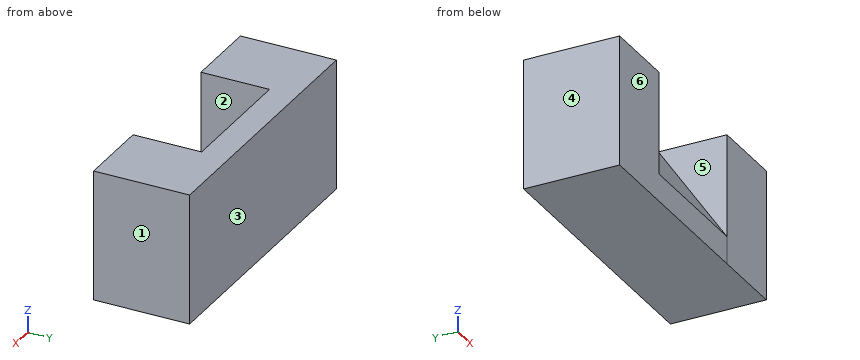
from build123d import *

# Parameters (mm, degrees)
F0_W     = 34.925
F0_H     = 60.325
F1_DEPTH = 44.45
F3_DEPTH = 60.325
F5_DEPTH = 34.925


with BuildPart() as f1:
    # F0 (on Front) → F1 (new body)
    with BuildSketch(Plane.XZ):
        with Locations((-46.881634, -30.1625)):
            Rectangle(F0_W, F0_H)
    extrude(amount=F1_DEPTH)

    # F2 (on face) → F3 (join)
    with BuildSketch(Plane.YZ.offset(-29.419134)):
        Polygon((-44.45, -47.625), (-44.45, -60.325), (0, -60.325), (0, -47.625), (0, 0), (-12.7, 0), align=None)
    extrude(amount=F3_DEPTH)

    # F4 (on face) → F5 (join)
    with BuildSketch(Plane.YZ.offset(30.905866)):
        Polygon((-44.45, -47.625), (-12.7, 0), (-44.459421, 0), (-44.45, -60.325), align=None)
        Polygon((0, -60.325), (0, 0), (-12.7, 0), (-44.45, -47.625), (-44.45, -60.325), align=None)
    extrude(amount=F5_DEPTH)


solid = f1.part
Design review of the part built by this model. Coordinates are the model's own, in mm. Face numbers are marked on the shaded views. A direction names the side the tool comes from. Round coordinates to 2 decimals unless told otherwise and drop trailing zeros. Loops run counter-clockwise (first coordinate to the right, second up) from the corner with the lowest first, then second, coordinate; pieces in that order, holes last. Notation, with made-up numbers: M 77.25,46 L 87.25,46 A23 ccw 87.25,72 Z; hole C -39.75,35.5 d2. An arc over 180 degrees is marked long. Answer as a JSON object with one key per item and string values.
Item 1: Clearance check with flat-ended pins moving along their axes: P1, Ø2, axis at x = 4, z = -51.5, coming from the -Y side; P2, Ø4, axis at x = -34.5, y = -33, coming from the +Z side. State where each tip first meets the part, or that it passes through.
Answer sheet:
{"P1": "stops at y = -44.45", "P2": "stops at z = 0"}
Item 2: Wall thickness on L1, parallel to X at y = -33.5, z = -8; L2, parallel to Y at x = -45.5, z = -41: over which ranges is each line inside the solid? List them lowest first. Write a range as from..to.
Answer sheet:
{"L1": "x = -64.34..-29.42, 30.91..65.83", "L2": "y = -44.45..0"}
Item 3: We need section A-A on y = -14.5. Give the boundary of the cut face in (x, z) (3 decimals).
Answer sheet:
{"outline": "M -64.344,-60.325 L 65.831,-60.325 L 65.831,0 L 30.906,0 L 30.906,-2.7 L -29.419,-2.7 L -29.419,0 L -64.344,0 Z"}
Item 4: Machinability: for the marked faces 5 and 6, which of the approach directions +Z, -Z, +X, -X, +Y, -Y give a long, thin tool a straight path to every point of the face, cutting with its end or side? Answer none if there is none.
Answer sheet:
{"face 5": "+Z, -Y", "face 6": "+Z, -Z, +X, -X, -Y"}
Item 5: The part is to be moulded in two halves that separate along X. For the marked faces 1, 2, 3 and 4, say which applies: pulls with the +X half, pulls with the -X half, needs draft (parallel to the pull), parting line crosses it, or undercut.
Answer sheet:
{"face 1": "pulls with the +X half", "face 2": "undercut", "face 3": "needs draft", "face 4": "pulls with the -X half"}
Item 6: We need section C-C on z = -41. Give the boundary of the cut face in (x, y), and give its area (3 significant figures).
Answer sheet:
{"outline": "M -64.34,-44.45 L -29.42,-44.45 L -29.42,-40.03 L 30.91,-40.03 L 30.91,-44.45 L 65.83,-44.45 L 65.83,0 L -64.34,0 Z", "area": "5,520 mm^2"}
Item 7: We need section B-B on x = 8. Give the boundary of the cut face in (y, z) (3 decimals), and give its area (3 significant figures).
Answer sheet:
{"outline": "M -44.45,-60.325 L 0,-60.325 L 0,0 L -12.7,0 L -44.45,-47.625 Z", "area": "1,930 mm^2"}
